Source: three-view drawing plus pictorial views. Frame: mm from the lowest corner of the part. Coordinates: 2 decimals unless noted, no trailing zeros. Loops run counter-clockwise (first coordinate to the right, second up) from the corner with the lowest first, then second, coordinate; pieces in that order, holes last. Notation, with made-up numbers: M -6.5,17 L 17.5,17 A7 ccw 17.5,23 Z; hole C 35,72 d9. An arc over 180 degrees is marked long. Use a Markdown table: item, result. Add a question column.
1. Section C-C on z = 7. Output: boundary loops of the cut face in (x, y) (3 decimals).
2. Line query: L1, parallel to Z at x = 0.75, y = 25.5; L2, parallel to Z at x = 0.95, y = 48; L3, parallel to Y at x = 2.35, z = 31. Output: solid intervals per line, ascending. Write a range as [from, to].
3. Pin query (flat end, axial travel): pin 1 (7.5 mm diameter, centred on y = 28.575, z = 9.525, fed in from +X). Return the tip coordinate at first contact, or that it passes through.
4. Section A-A on z = 30.5. Output: boundary loops of the cut face in (x, y) (3 decimals).
5. Section B-B on y = 27. State how many separate pieces and enclosed holes the cut face has, then the cut area to 3 significant figures.
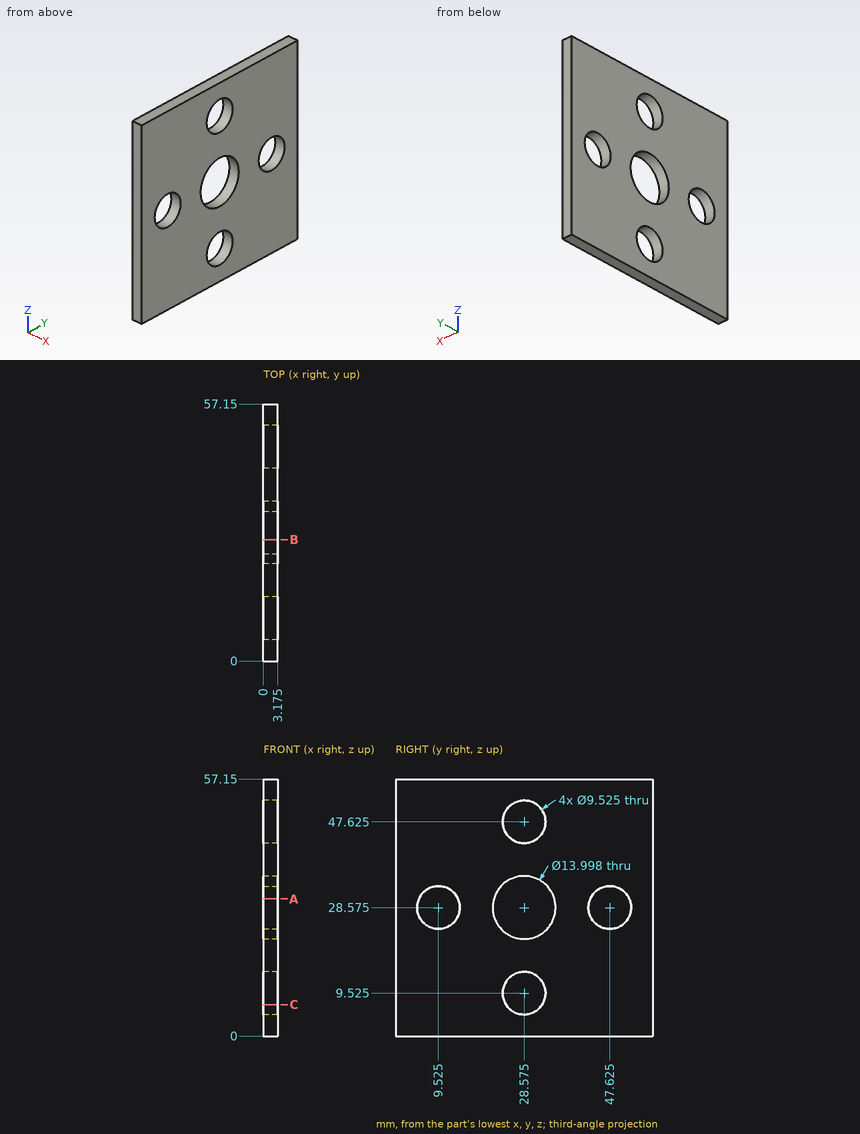
Answers below:
| question | item | result |
|---|---|---|
| 1 | outline | M 0,0 L 3.175,0 L 3.175,24.537 L 0,24.537 Z; M 0,32.613 L 3.175,32.613 L 3.175,57.15 L 0,57.15 Z |
| 2 | L1 | z = [0, 5.89], [13.16, 22.29], [34.86, 43.99], [51.26, 57.15] |
| 2 | L2 | z = [0, 23.83], [33.32, 57.15] |
| 2 | L3 | y = [0, 5.43], [13.62, 22.01], [35.14, 43.53], [51.72, 57.15] |
| 3 | pin 1 | passes through |
| 4 | outline | M 0,0 L 3.175,0 L 3.175,5.169 L 0,5.169 Z; M 0,13.881 L 3.175,13.881 L 3.175,21.846 L 0,21.846 Z; M 0,35.304 L 3.175,35.304 L 3.175,43.269 L 0,43.269 Z; M 0,51.981 L 3.175,51.981 L 3.175,57.15 L 0,57.15 Z |
| 5 | separate pieces | 4 |
| 5 | enclosed holes | 0 |
| 5 | area | 81.1 mm² |
